Autodesk Inventor part; units mm, degrees
ref_plane "YZ Plane" through (0, 0, 0) normal (1, 0, 0) x (0, 1, 0)
ref_plane "XZ Plane" through (0, 0, 0) normal (0, 1, 0) x (-1, 0, 0)
ref_plane "XY Plane" through (0, 0, 0) normal (0, 0, 1) x (1, 0, 0)
sketch "Sketch1" plane through (0, 0, 0) normal (0, 1, 0) x (-1, 0, 0)
  line L0 (0, 0) -> (67.31, 0)
  line L1 (67.31, 0) -> (67.31, -40.005)
  line L2 (67.31, -40.005) -> (0, -40.005)
  line L3 (0, -40.005) -> (0, 0)
  dimension "d0" = 40.005
  dimension "d1" = 67.31
extrude "Extrusion1" add sketch "Sketch1" along normal blind 3.175
sketch "Sketch2" plane through (0, 3.175, 0) normal (0, 1, 0) x (1, 0, 0)
  circle A0 centre (-13.97, 12.7) radius 4.445
  line L0 (0, 0) -> (0, 40.005)
  line L1 (-67.31, 0) -> (0, 0)
  dimension "d4" = 13.97
  dimension "d5" = 12.7
  dimension "d28" = 8.89
extrude "Extrusion2" cut sketch "Sketch2" against normal blind 6.35
sketch "Sketch3" plane through (0, 0, 0) normal (0, -1, 0) x (1, 0, 0)
  line L0 (0, -40.005) -> (-67.31, -40.005)
  line L1 (-67.31, 0) -> (0, 0)
  line L2 (-67.31, -40.005) -> (-51.435, -40.005)
  line L3 (-51.435, -40.005) -> (-51.435, 0)
  line L4 (-51.435, 0) -> (-67.31, 0)
  line L5 (-67.31, 0) -> (-67.31, -40.005)
  dimension "d8" = 15.875
extrude "Extrusion3" add sketch "Sketch3" along normal blind 16.51
sketch "Sketch4" plane through (-67.31, 3.175, -40.005) normal (-1, 0, 0) x (0, 0, 1)
  line L0 (40.005, -19.685) -> (0, -19.685)
  circle A0 centre (20.0025, -19.685) radius 6.35
  point P0 (40.005, -3.175)
  point P1 (13.6525, -19.685)
  point P2 (26.3525, -19.685)
  dimension "d11" = 12.7
extrude "Extrusion4" cut sketch "Sketch4" against normal blind 6.35 contours L0 A0 picked at (22.0577, -19.1784)
sketch "Sketch5" plane through (-60.96, 3.175, -40.005) normal (-1, 0, 0) x (0, 0, 1)
  line L0 (26.3525, -19.685) -> (13.6525, -19.685)
  line L1 (20.0025, -19.685) -> (20.0025, -3.683)
  circle A0 centre (20.0025, -3.683) radius 3.175
  arc A1 (26.3525, -19.685) -> (13.6525, -19.685) centre (20.0025, -19.685) ccw
  line L2 (24.765, -15.4849) -> (15.24, -15.4849)
  line L3 (24.765, -15.4849) -> (23.1501, -3.267)
  line L4 (15.24, -15.4849) -> (16.8549, -3.267)
  point P0 (40.005, -3.175)
  dimension "d14" = 16.002
  dimension "d15" = 6.35
  dimension "d16" = 9.525
extrude "Extrusion5" cut sketch "Sketch5" along normal blind 2.54 contours A1 L1 A0 L3 | A1 L4 A0 L1 | A0
sketch "Sketch6" plane through (0, 3.175, 0) normal (0, 1, 0) x (1, 0, 0)
  circle A0 centre (-55.88, 30.48) radius 2.1828
  circle A1 centre (-55.88, 11.43) radius 2.1828
  line L0 (-67.31, 40.005) -> (-67.31, 0)
  line L1 (-67.31, 0) -> (0, 0)
  line L2 (0, 40.005) -> (-67.31, 40.005)
  dimension "d19" = 4.3656
  dimension "d20" = 4.3656
  dimension "d21" = 11.43
  dimension "d22" = 11.43
  dimension "d23" = 19.05
  dimension "d32" = 9.525
extrude "Extrusion6" cut sketch "Sketch6" against normal blind 25.4
fillet "Fillet1" radius 1.27 9 edges at (0, 0, -20.0025) (-25.7175, 0, 0) (-25.7175, 0, -40.005) (-51.435, -8.255, 0) (0, 1.5875, 0) (0, 1.5875, -40.005) (-67.31, -6.6675, -40.005) (-51.435, -8.255, -40.005) (-67.31, -6.6675, 0)
sketch "Sketch7" plane through (-67.31, -16.51, -20.0025) normal (-1, 0, 0) x (0, 0, 1)
  arc A0 (4.7625, 4.2001) -> (-4.7625, 4.2001) centre (0, 0) ccw
  circle A1 centre (0, 0) radius 4.7625
  point P0 (20.0025, 16.51)
  dimension "d29" = 9.525
extrude "Extrusion7" cut sketch "Sketch7" against normal blind 25.4
properties part number "SwerveDriveBracket_A"
The model under review builds one solid part; all positions refer to its coordinate system, in mm. A direction names the side the tool comes from. Round coordinates to 2 decimals unless told otherwise and drop trailing zeros. Loops run counter-clockwise (first coordinate to the right, second up) from the corner with the lowest first, then second, coordinate; pieces in that order, holes last. Notation, with made-up numbers: (29.25, 21.25) -> (47.25, 21.25) arc R9 ccw to (47.25, 25.25) -> close; hole circle Ø8 at (67.25, 5). An arc over 180 degrees is marked (long way). Answer in a Markdown table with one row per item.
1) Consider section D-D, the plane y = -1. Write out the cut boundary in (x, z) (3 decimals), plus the area to 3 significant figures.
Taken from the geometry:
| item | result |
|---|---|
| outline | (-67.31, -38.735) arc R1.27 ccw to (-66.04, -40.005) -> (-52.705, -40.005) arc R1.27 ccw to (-51.435, -38.735) -> (-51.435, -1.27) arc R1.27 ccw to (-52.705, 0) -> (-66.04, 0) arc R1.27 ccw to (-67.31, -1.27) -> close; hole (-63.5, -23.27) -> (-60.96, -23.27) -> (-60.96, -16.735) -> (-63.5, -16.735) -> close; hole circle Ø4.366 at (-55.88, -30.48); hole circle Ø4.366 at (-55.88, -11.43) |
| area | 587 mm² |
2) Consider section A-A, the plane x = -13.97. Write out the cut boundary in (y, z) (3 decimals).
Taken from the geometry:
| item | result |
|---|---|
| outline | (0, -38.735) arc R1.27 ccw to (1.27, -40.005) -> (3.175, -40.005) -> (3.175, -17.145) -> (0, -17.145) -> close; (0, -8.255) -> (3.175, -8.255) -> (3.175, 0) -> (1.27, 0) arc R1.27 ccw to (0, -1.27) -> close |
3) For pin 1 Ø1.5 at (y, z) = (-12, -12.5) entering from +X (3 decimals); pin 2 Ø3.5 at (x, z) = (-55.88, -11.43) entering from +Y; pin 3 Ø5 at (x, z) = (-11.5, -29.5) entering from -Y; pin 4 Ø4 at (x, y) = (-9, -1.5) entering from +Z, all flat-tipped, find the tip position at first contact; note any pin that passes through.
Taken from the geometry:
| item | result |
|---|---|
| pin 1 | stops at x = -51.435 |
| pin 2 | passes through |
| pin 3 | stops at y = 0 |
| pin 4 | stops at z = -0.26 |
4) Consider section B-B, the plane z = -30.48. Write out the cut boundary in (x, y) (3 decimals), plus the area to 3 significant figures.
Taken from the geometry:
| item | result |
|---|---|
| outline | (-67.31, -16.51) -> (-58.063, -16.51) -> (-58.063, 3.175) -> (-67.31, 3.175) -> close; (-53.697, -16.51) -> (-51.435, -16.51) -> (-51.435, 0) -> (-1.27, 0) arc R1.27 ccw to (0, 1.27) -> (0, 3.175) -> (-53.697, 3.175) -> close |
| area | 390 mm² |
5) Tool access review of faces 1 (the cylindrical face through (-64.89, -10.16, -19.86)), 2 (the flat face through (-51.435, -8, -20)), 3 (the cylindrical face through (-26.63, 0.36, -39.62)), 4 (the cylindrical face through (-51.8, -7.74, -0.38)): name each direction out of +Z, -Z, +X, -X, +Y, -Y from which nothing blocks a thin tool from reaching the whole face with its end or side.
Taken from the geometry:
| item | result |
|---|---|
| face 1 | -X, -Y |
| face 2 | +Z, -Z, +X, -Y |
| face 3 | -Z, +X, -Y |
| face 4 | +Z, +X, -Y |
6) Consider section C-C, the plane x = -55.88. Write out the cut boundary in (y, z) (1 decimal).
Taken from the geometry:
| item | result |
|---|---|
| outline | (-16.5, -40) -> (3.2, -40) -> (3.2, -32.7) -> (-16.5, -32.7) -> close; (-16.5, -28.3) -> (3.2, -28.3) -> (3.2, -13.6) -> (-16.5, -13.6) -> (-16.5, -15.2) arc R4.8 cw to (-16.5, -24.8) -> close; (-16.5, -9.2) -> (3.2, -9.2) -> (3.2, 0) -> (-16.5, 0) -> close |
7) Draft analysis for pull direction X (two halves, no side actions). For faces 5 (the cylindrical face through (-27.348, 0.362, -0.382)), 6 (the cylindrical face through (-66.948, -6.53, -0.382)), 7 (the flat face through (-62.21, -6.29, -23.97)), 8 (the flat face through (-62.212, -6.286, -16.036)), state which applies: pulls with the +X half, pulls with the -X half, needs draft (parallel to the pull), parting line crosses it, or undercut.
Taken from the geometry:
| item | result |
|---|---|
| face 5 | needs draft |
| face 6 | pulls with the -X half |
| face 7 | undercut |
| face 8 | undercut |
8) Wall thickness on line 1 along Z through (x, y) = (-55.88, -6.5) (3 decimals); line 2 along X through (y, z) = (2.2, -12.7) (3 decimals); line 3 along X through (y, z) = (-6, -5.5) (3 decimals): over which ranges is each line inside the solid? List them lowest first.
Taken from the geometry:
| item | result |
|---|---|
| line 1 | z = -40.005 to -32.663, -28.297 to -13.613, -9.247 to 0 |
| line 2 | x = -67.31 to -57.655, -54.105 to -18.415, -9.525 to 0 |
| line 3 | x = -67.31 to -51.435 |
